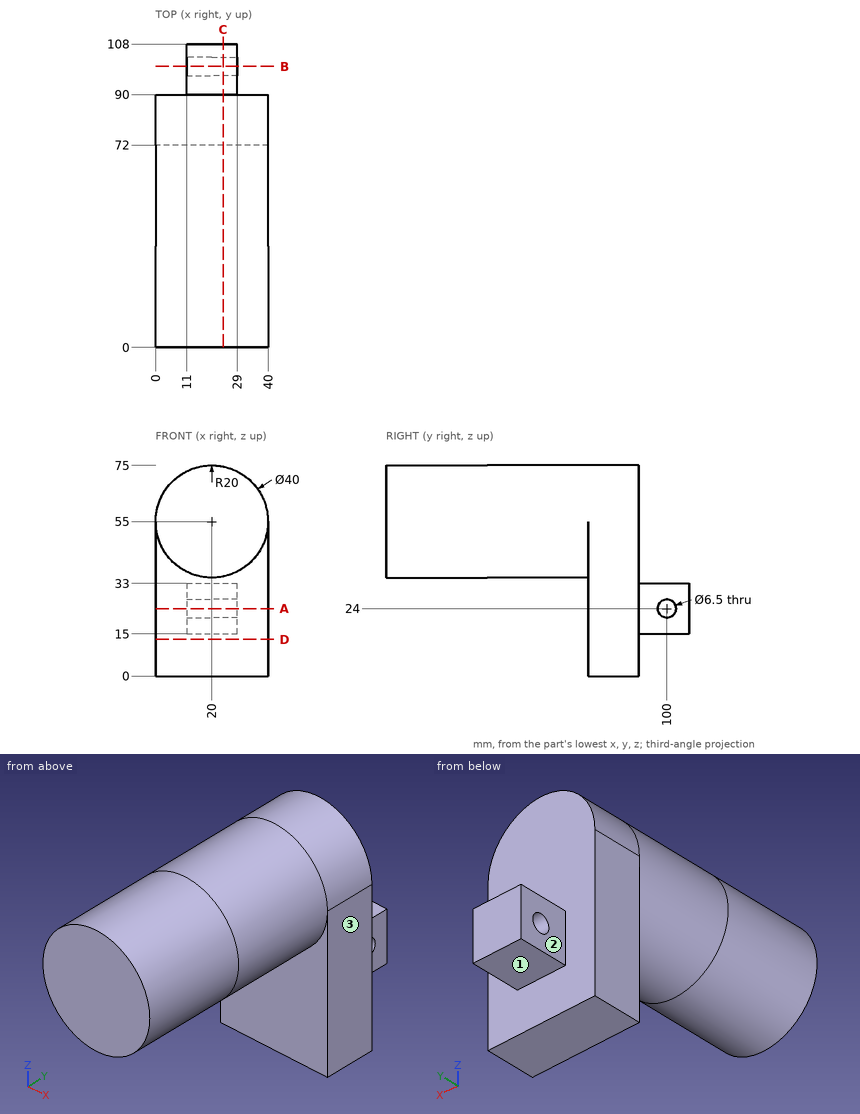
Answer from the drawing. Dimensions are ordinates in mm from the lowest x, y and z of the part. A direction names the side the tool comes from. Round coordinates to 2 decimals unless told otherwise and drop trailing zeros. Write each loop counter-clockwise with the first axis right and the second up, starting at its lowest first coordinate (ties: lowest second). Pieces come first, ordered by that corner, then holes. Notation, with made-up numbers: (-0.5, -4.75) -> (11.5, -4.75) arc R11 ccw to (11.5, 6.25) -> close; hole circle Ø8 at (-34.75, 36). An arc over 180 degrees is marked (long way). Write each question's results on one line, items separated by ' | '.
1) The part is cut by section A-A (z = 24). Write down the section's boundary in (x, y), and give its area (3 significant figures).
Findings:
outline: (0, 72) -> (40, 72) -> (40, 90) -> (29, 90) -> (29, 96.75) -> (11, 96.75) -> (11, 90) -> (0, 90) -> close; (11, 103.25) -> (29, 103.25) -> (29, 108) -> (11, 108) -> close | area: 927 mm²
2) The part is cut by section D-D (z = 13). Write down the section's boundary in (x, y).
Findings:
outline: (0, 72) -> (40, 72) -> (40, 90) -> (0, 90) -> close
3) Which of the six approach directions +Z, -Z, +X, -X, +Y, -Y give full straight-line access (tool end or side, diameter ignored) to the marked faces 1, 2 and 3?
Findings:
face 1: -Z, +X, -X, +Y | face 2: +Z, -Z, -X, +Y | face 3: +Z, -Z, +X, +Y, -Y
4) The part is cut by section B-B (y = 100). Write down the section's boundary in (x, z), and give its area (3 significant figures).
Findings:
outline: (11, 15) -> (29, 15) -> (29, 20.75) -> (11, 20.75) -> close; (11, 27.25) -> (29, 27.25) -> (29, 33) -> (11, 33) -> close | area: 207 mm²
5) Consider line 1 along Z through (x, y) = (25, 100); line 2 along Y through (x, z) = (24.75, 24); line 3 along Z through (x, y) = (20.5, 5.5). Determine where each line is inside the solid, lowest interval first. Write a range as [from, to].
Findings:
line 1: z = [15, 20.75], [27.25, 33] | line 2: y = [72, 96.75], [103.25, 108] | line 3: z = [35.01, 74.99]
6) The part is cut by section C-C (x = 24). Write down the section's boundary in (y, z).
Findings:
outline: (0, 35.4) -> (72, 35.4) -> (72, 0) -> (90, 0) -> (90, 15) -> (108, 15) -> (108, 33) -> (90, 33) -> (90, 74.6) -> (0, 74.6) -> close; hole circle Ø6.5 at (100, 24)
7) Flat-ended cylindrical pins translate along their axes: pin 1 (12 mm diameter, centred on x = 16, z = 23, fed in from -Y); pin 2 (20 mm diameter, centred on x = 18, y = 100.5, fed in from +Z); pin 3 (3 mm diameter, centred on y = 90, z = 61, fed in from +X). Find the tip coordinate at first contact, or state that the pin passes through.
Findings:
pin 1: stops at y = 72 | pin 2: stops at z = 33 | pin 3: stops at x = 39.49
